```python
from build123d import *

# Parameters (mm, degrees)
F1_DEPTH = 4
F2_DEPTH = 14
F0_W     = 7
F0_H     = 7
F3_DEPTH = 25


with BuildPart() as f1:
    # F0 (on Top) → F1 (new body)
    with BuildSketch(Plane.XY):
        Polygon((7, 1.6), (40, 1.6), (40, 34.6), (38.8, 34.6), (38.8, 53.8), (1.2, 53.8), (1.2, 34.6), (0, 34.6), (0, 29.6), (7, 29.6), (7, 22.6), align=None)
    extrude(amount=F1_DEPTH)

    # F0 (on Top) → F2 (join)
    with BuildSketch(Plane.XY):
        Polygon((0, 22.6), (0, 0), (40, 0), (40, 1.6), (7, 1.6), (7, 22.6), align=None)
        Polygon((38.8, 34.6), (40, 34.6), (40, 55), (0, 55), (0, 34.6), (1.2, 34.6), (1.2, 53.8), (38.8, 53.8), align=None)
    extrude(amount=F2_DEPTH)

    # F0 (on Top) → F3 (join)
    with BuildSketch(Plane.XY):
        with Locations((3.5, 26.1)):
            Rectangle(F0_W, F0_H)
    extrude(amount=F3_DEPTH)


solid = f1.part
```
Input: part model. Units: mm. Frame: model coordinates. A direction names the side the tool comes from. Coordinates: 2 decimals unless noted, no trailing zeros. Loops run counter-clockwise (first coordinate to the right, second up) from the corner with the lowest first, then second, coordinate; pieces in that order, holes last. Notation, with made-up numbers: (26, 37.25) - (73, 37.25) arc R24 ccw to (73, 71.25) - close; hole circle Ø2 at (47.25, 62.25). An arc over 180 degrees is marked (long way). Answer in a Markdown table with one row per item.
(1) Set-up query: faces 1 (the face through (6.6, 8.8, 14)), 2 (the face through (20, 53.8, 9)), 3 (the face through (7, 19, 10)), 4 (the face through (3, 29.6, 14)). Return all of +Z, -Z, +X, -X, +Y, -Y with unobstructed straight access to the full face (end or side cutting, diameter ignored); none if empty.
Model answer:
| item | result |
|---|---|
| face 1 | +Z, +X, -X, -Y |
| face 2 | +Z |
| face 3 | +Z, +X |
| face 4 | +Z, +X, -X |
(2) Pin query (flat end, axial travel): P1, Ø1, axis at x = 19, y = 41.5, coming from the +Z side; P2, Ø11.5, axis at x = 16.5, y = 7, coming from the +Z side; P3, Ø2, axis at x = 4, z = 18.5, coming from the +Y side. Return the tip coordinate at first contact, or that it passes through.
Model answer:
| item | result |
|---|---|
| P1 | stops at z = 4 |
| P2 | stops at z = 14 |
| P3 | stops at y = 29.6 |
(3) Cut plane A-A on z = 5.5. Output: boundary loops of the cut face in (x, y).
Model answer:
| item | result |
|---|---|
| outline | (0, 0) - (40, 0) - (40, 1.6) - (7, 1.6) - (7, 29.6) - (0, 29.6) - close; (0, 34.6) - (1.2, 34.6) - (1.2, 53.8) - (38.8, 53.8) - (38.8, 34.6) - (40, 34.6) - (40, 55) - (0, 55) - close |
(4) Cut plane B-B on y = 18. Output: boundary loops of the cut face in (x, z), plus the area to 3 significant figures.
Model answer:
| item | result |
|---|---|
| outline | (0, 0) - (40, 0) - (40, 4) - (7, 4) - (7, 14) - (0, 14) - close |
| area | 230 mm² |
(5) Material intervals for L1, parallel to Y at x = 11.5, z = 6.5; L2, parallel to Z at x = 37, y = 27; L3, parallel to X at y = 26.5, z = 7, sorted ascending. Write a range as from..to.
Model answer:
| item | result |
|---|---|
| L1 | y = 0..1.6, 53.8..55 |
| L2 | z = 0..4 |
| L3 | x = 0..7 |
(6) Cut plane C-C on x = 5. Output: boundary loops of the cut face in (y, z), plus the area to 3 significant figures.
Model answer:
| item | result |
|---|---|
| outline | (0, 0) - (55, 0) - (55, 14) - (53.8, 14) - (53.8, 4) - (29.6, 4) - (29.6, 25) - (22.6, 25) - (22.6, 14) - (0, 14) - close |
| area | 605 mm² |
(7) Mould query, pull axis Y, two halves, no side actions, for faces 5 (the face through (24, 1.6, 9)), 6 (the face through (3, 22.6, 19)), 7 (the face through (20, 55, 7)), 8 (the face through (0, 27, 7)). Classes: pulls with the +Y half, pulls with the -Y half, needs draft (parallel to the pull), parting line crosses it, or undercut.
Model answer:
| item | result |
|---|---|
| face 5 | undercut |
| face 6 | pulls with the -Y half |
| face 7 | pulls with the +Y half |
| face 8 | needs draft |
(8) Cut plane D-D on z = 18.5. Output: boundary loops of the cut face in (x, y).
Model answer:
| item | result |
|---|---|
| outline | (0, 22.6) - (7, 22.6) - (7, 29.6) - (0, 29.6) - close |
